Build history of the part. All positions in model axes, mm. A direction names the side the tool comes from. Coordinates: 2 decimals unless noted, no trailing zeros. Write each loop counter-clockwise with the first axis right and the second up, starting at its lowest first coordinate (ties: lowest second). Pieces come first, ordered by that corner, then holes.
from build123d import *

# Parameters (mm, degrees)
SKETCH_1_R      = 2.4
EXTRUDE_1_DEPTH = 2.5
SKETCH_3_R      = 3.5
EXTRUDE_2_DEPTH = 0.5


with BuildPart() as part:
    # Эскиз1 → Бобышка-Вытянуть1 (new body)
    with BuildSketch(Plane(origin=(0, 0, 0), x_dir=(1, 0, 0), z_dir=(0, 1, 0))):
        with Locations(Location((0, 0, 0), (0, 0, 270))):
            Circle(SKETCH_1_R)
    extrude(amount=EXTRUDE_1_DEPTH)

    # Эскиз2 → Вырез-Повернуть1 (revolve, cut)
    with BuildSketch(Plane(origin=(0, 0, 0), x_dir=(0, 0, -1), z_dir=(1, 0, 0))):
        with BuildLine():
            Line((0, 2.5), (0, 2.149039298))
            ThreePointArc((0, 2.149039298), (1.212762695, 2.237243589), (2.4, 2.5))
            Line((2.4, 2.5), (0, 2.5))
        make_face()
    revolve(axis=Axis((0, 2.5, 0), (0, 1, 0)), mode=Mode.SUBTRACT)

    # Эскиз3 → Бобышка-Вытянуть2 (add)
    with BuildSketch(Plane.XZ):
        with Locations(Location((0, 0, 0), (0, 0, 270))):
            Circle(SKETCH_3_R)
    extrude(amount=-EXTRUDE_2_DEPTH)


solid = part.part
(1) Slice it at B-B, the plane x = 0. List the corners of the cut face in (y, z), and give its area (3 significant figures).
(2) Slice it at C-C, the plane y = 1. List the corners of the cut face in (x, z), and give its area (3 significant figures).
(3) Slice it at D-D, the plane z = 2. List the corners of the cut face in (x, y).
(4) Slice it at A-A, the plane z = 0. List the corners of the cut face in (x, y), and give its area (3 significant figures).
(5) Flat gauge pin, fed straight in: P1, Ø1, axis at y = 1.5, z = 2.5, coming from the +X side. Where does the tip first touch, or does it go through?
(6) Probe L1, parallel to Y at x = -2, z = 1.75; L2, parallel to Z at x = 0, y = 1.85; L3, parallel to X at y = 2.25, z = -1.5. List the from-to ranges inside material, lowest first.
(7) 3-axis set-ups, long thin cutter, end or side, ignore diameter. For faces 1 (the cylindrical face through (-3.417, 0.246, 0.759)), 2 (the cylindrical face through (2.024, 1.486, 1.29)): which of +Z, -Z, +X, -X, +Y, -Y reach the whole face in a straight line?
Results:
1. outline: (0, -3.5) - (0.5, -3.5) - (0.5, -2.4) - (2.5, -2.4) arc R8.38 cw to (2.5, 2.4) - (0.5, 2.4) - (0.5, 3.5) - (0, 3.5) - close
1. area: 12.0 mm2
2. outline: circle Ø4.8 at (0, 0)
2. area: 18.1 mm2
3. outline: (-2.87, 0) - (2.87, 0) - (2.87, 0.5) - (1.33, 0.5) - (1.33, 2.5) arc R8.14 cw to (-1.33, 2.5) - (-1.33, 0.5) - (-2.87, 0.5) - close
4. outline: (-3.5, 0) - (3.5, 0) - (3.5, 0.5) - (2.4, 0.5) - (2.4, 2.5) arc R8.38 cw to (-2.4, 2.5) - (-2.4, 0.5) - (-3.5, 0.5) - close
4. area: 12.0 mm2
5. P1: stops at x = 1.33
6. L1: y = 0 to 0.5
6. L2: z = -2.4 to 2.4
6. L3: x = -1.87 to 1.87
7. face 1: +Y, -Y
7. face 2: +Y
